CAD build for the part. Positions are in the model's coordinates, mm. Face numbers are marked on the shaded views. Coordinates: 2 decimals unless noted, no trailing zeros. Loops run counter-clockwise (first coordinate to the right, second up) from the corner with the lowest first, then second, coordinate; pieces in that order, holes last. Notation, with made-up numbers: (42.5, 44) -> (52.5, 44) arc R25 ccw to (52.5, 59) -> close; hole circle Ø5 at (-4.75, -40). An arc over 180 degrees is marked (long way). Answer as CSV lines item,"result". Start each with the question number.
from build123d import *

# Parameters (mm, degrees)
SKETCH1_R               = 5
BOSS_EXTRUDE1_DEPTH     = 35.4
SKETCH2_R               = 1
CUT_EXTRUDE1_DEPTH      = 6
CUT_EXTRUDE1_DEPTH_BACK = 6
SKETCH3_OUTSIDE_W       = 19.624
SKETCH3_OUTSIDE_H       = 19.624
SKETCH3_OUTSIDE_R       = 3.5
CUT_EXTRUDE2_DEPTH      = 10


with BuildPart() as part:
    # Sketch1 → Boss-Extrude1 (new body)
    with BuildSketch(Plane.XY):
        Circle(SKETCH1_R)
    extrude(amount=BOSS_EXTRUDE1_DEPTH)

    # Sketch2 → Cut-Extrude1 (cut, two sides)
    with BuildSketch(Plane(origin=(0, 0, 0), x_dir=(0, 0, -1), z_dir=(1, 0, 0))) as cut_extrude1_sk:
        with Locations((-2.031417136, 0)):
            Circle(SKETCH2_R)
    extrude(amount=CUT_EXTRUDE1_DEPTH, mode=Mode.SUBTRACT)
    extrude(cut_extrude1_sk.sketch, amount=-CUT_EXTRUDE1_DEPTH_BACK, mode=Mode.SUBTRACT)

    # Sketch3 outside → Cut-Extrude2 (cut)
    with BuildSketch(Plane(origin=(0, 0, 0), x_dir=(-1, 0, 0), z_dir=(0, 0, -1))):
        Rectangle(SKETCH3_OUTSIDE_W, SKETCH3_OUTSIDE_H)
        Circle(SKETCH3_OUTSIDE_R, mode=Mode.SUBTRACT)
    extrude(amount=-CUT_EXTRUDE2_DEPTH, mode=Mode.SUBTRACT)


solid = part.part
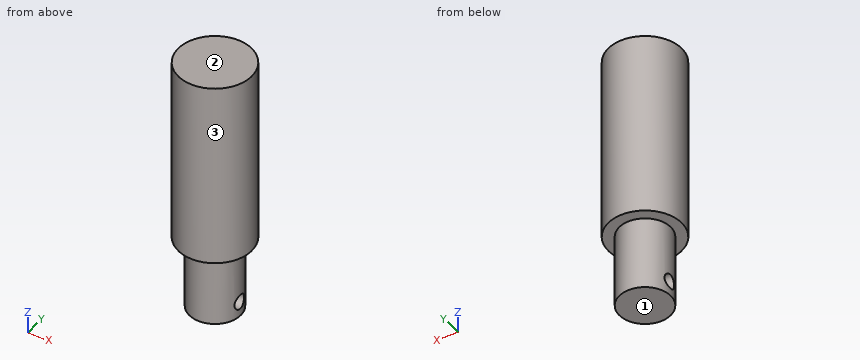
Item 1: Saw through at B-B (x = 0). Write the cut outline in (y, z).
Item 2: Flat gauge pins, fed straight in: pin 1 Ø5 at (x, z) = (1.5, 7) entering from +Y; pin 2 Ø2 at (x, z) = (-1.5, 27.5) entering from -Y; pin 3 Ø1 at (x, z) = (3.5, 12) entering from -Y. Where does each tip first touch, or does it go through?
Item 3: Two-plate mould, pull along Z, no slides. Class the marked faces 1, 2 and 3: pulls with the +Z half, pulls with the -Z half, needs draft (parallel to the pull), parting line crosses it, or undercut.
Item 4: Wall check: probe 1 along Z at (x, y) = (-1.25, 0); probe 2 along Z at (x, y) = (-2, 3); probe 3 along Z at (x, y) = (-2.5, -0.5). Give the ranges that are in metal, low to high.
Item 5: Saw through at A-A (y = 0). Write the cut outline in (x, z), plus the area to 3 significant figures.
Item 6: Saw through at C-C (y = 2). Write the cut outline in (x, z), plus the area to 3 significant figures.
Item 7: Saw through at D-D (z = 33). Write the cut outline in (x, y), plus the area to 3 significant figures.
Geometry check:
1,outline,"(-5, 10) -> (-3.5, 10) -> (-3.5, 0) -> (3.5, 0) -> (3.5, 10) -> (5, 10) -> (5, 35.4) -> (-5, 35.4) -> close; hole circle Ø2 at (0, 2.03)"
2,pin 1,"y = 3.5"
2,pin 2,"y = -4.97"
2,pin 3,"y = -4"
3,face 1,"pulls with the -Z half"
3,face 2,"pulls with the +Z half"
3,face 3,"needs draft"
4,probe 1,"0 to 1.03, 3.03 to 35.4"
4,probe 2,"10 to 35.4"
4,probe 3,"0 to 1.17, 2.9 to 35.4"
5,outline,"(-5, 10) -> (-3.5, 10) -> (-3.5, 3.03) -> (3.5, 3.03) -> (3.5, 10) -> (5, 10) -> (5, 35.4) -> (-5, 35.4) -> close; (-3.5, 0) -> (3.5, 0) -> (3.5, 1.03) -> (-3.5, 1.03) -> close"
5,area,"310 mm2"
6,outline,"(-4.58, 10) -> (-2.87, 10) -> (-2.87, 0) -> (2.87, 0) -> (2.87, 10) -> (4.58, 10) -> (4.58, 35.4) -> (-4.58, 35.4) -> close"
6,area,"290 mm2"
7,outline,"circle Ø10 at (0, 0)"
7,area,"78.5 mm2"
